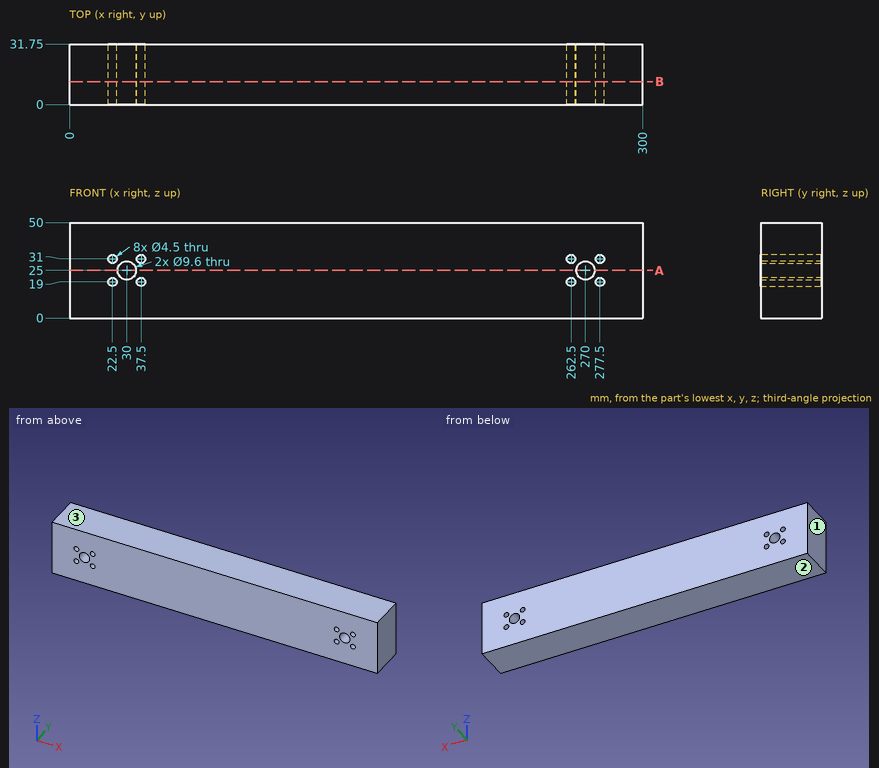
Design review of the part shown in the three views and the two pictorial views. Dimensions are in mm from the part's minimum x, y and z. Round coordinates to 2 decimals unless told otherwise and drop trailing zeros. Write each loop counter-clockwise with the first axis right and the second up, starting at its lowest first coordinate (ties: lowest second). Pieces come first, ordered by that corner, then holes.
1) Take a section at B-B on y = 12. State how many separate pieces and enclosed holes the cut face has, then the cut area to 3 significant figures.
Answer below:
separate pieces: 1
enclosed holes: 10
area: 14,700 mm2
2) Insertion check: pin 1 Ø8.5 at (x, z) = (30, 25) entering from -Y. The pin has a flat end and moves straight along its axis. Give the tip position at first contact, or say it passes through.
Answer below:
pin 1: passes through
3) For line 1 along X through (y, z) = (20, 19); line 2 along Z through (x, y) = (262.5, 24); line 3 along X through (y, z) = (26.5, 26), list the stretches that pass through material, from the lowest coordinate up.
Answer below:
line 1: x = 0 to 20.25, 24.75 to 35.25, 39.75 to 260.25, 264.75 to 275.25, 279.75 to 300
line 2: z = 0 to 16.75, 21.25 to 28.75, 33.25 to 50
line 3: x = 0 to 25.31, 34.69 to 265.31, 274.69 to 300
4) Take a section at A-A on z = 25. Give the boundary of the cut face in (x, y), then the cut area to 3 significant figures.
Answer below:
outline: (0, 0) - (25.2, 0) - (25.2, 31.75) - (0, 31.75) - close; (34.8, 0) - (265.2, 0) - (265.2, 31.75) - (34.8, 31.75) - close; (274.8, 0) - (300, 0) - (300, 31.75) - (274.8, 31.75) - close
area: 8,920 mm2
5) Mouldability with a two-part tool opening along Z and no side actions: class the marked faces 1, 2 and 3 as +Z half, -Z half, draft (parallel to the pull), parting line (faces both ways), or undercut.
Answer below:
face 1: draft
face 2: -Z half
face 3: +Z half
